Could you check a few things on this model? Use its own coordinates, in mm. Round coordinates to 2 decimals unless told otherwise and drop trailing zeros. Write each loop counter-clockwise with the first axis right and the second up, starting at its lowest first coordinate (ties: lowest second). Pieces come first, ordered by that corner, then holes. Notation, with made-up numbers: (75.5, 14) -> (110.5, 14) arc R13 cw to (110.5, 34) -> close; hole circle Ø1 at (5.25, -19.75). An arc over 180 degrees is marked (long way). One line per question, with ' | ' between items. Start each with the question number.
1. Thinking about a two-plate mould opening in Y: for faces 1 (the flat face through (-1, -1, 6)), 2 (the cylindrical face through (24.5, 7.1, 3)), 3 (the flat face through (-1, 35, 3)), which applies, released by +Y, released by -Y, zero draft, split by the parting line, or undercut?
2. If I drill on line 1 along Y through (x, z) = (-27, 2.35); line 2 along Y through (x, z) = (21.5, 2.3); line 3 along Y through (x, z) = (-26.5, 3.8), over which ranges is the centre line in solid material (lowest first)? Write a range as [from, to].
3. Imagine slicing it at D-D, the plane y = 7. List the corners of the cut face in (x, z) for me, and give its area (3 significant figures).
4. Imagine slicing it at A-A, the plane z = 3. List the corners of the cut face in (x, y) for me.
5. Imagine slicing it at C-C, the plane x = 0. List the corners of the cut face in (y, z) for me, and give its area (3 significant figures).
6. Imagine slicing it at B-B, the plane y = 30. List the corners of the cut face in (x, z) for me.
from build123d import *

# Parameters (mm, degrees)
SKETCH_1_W          = 80
SKETCH_1_H          = 60
SKETCH_1_R          = 7
EXTRUDE_1_DEPTH     = 6
SKETCH_2_R          = 3
SKETCH_2_R_2        = 2.555087711
CUT_EXTRUDE_1_DEPTH = 10


with BuildPart() as part:
    # 草图1 → 凸台-拉伸1 (new body)
    with BuildSketch(Plane.XY):
        with Locations((0, 5)):
            Rectangle(SKETCH_1_W, SKETCH_1_H)
        with Locations((0, 7)):
            Circle(SKETCH_1_R, mode=Mode.SUBTRACT)
    extrude(amount=EXTRUDE_1_DEPTH)

    # 草图2 → 切除-拉伸1 (cut)
    with BuildSketch(Plane(origin=(0, 0, 0), x_dir=(-1, 0, 0), z_dir=(0, 0, -1))):
        with Locations((-21.5, 7)):
            Circle(SKETCH_2_R)
        with Locations((26.5, 7)):
            Circle(SKETCH_2_R)
        with Locations((27, 30)):
            Circle(SKETCH_2_R_2)
        with Locations((27, -16)):
            Circle(SKETCH_2_R_2)
        with Locations((-25.052626778, -16)):
            Circle(SKETCH_2_R_2)
        with Locations((-25.052626778, 30)):
            Circle(SKETCH_2_R_2)
    extrude(amount=-CUT_EXTRUDE_1_DEPTH, mode=Mode.SUBTRACT)


solid = part.part
Geometry results:
1) face 1: zero draft | face 2: undercut | face 3: released by +Y
2) line 1: y = [-25, -18.56], [-13.44, 4.04], [9.96, 27.44], [32.56, 35] | line 2: y = [-25, 4], [10, 35] | line 3: y = [-25, -18.51], [-13.49, 4], [10, 27.49], [32.51, 35]
3) outline: (-40, 0) -> (-29.5, 0) -> (-29.5, 6) -> (-40, 6) -> close; (-23.5, 0) -> (-7, 0) -> (-7, 6) -> (-23.5, 6) -> close; (7, 0) -> (18.5, 0) -> (18.5, 6) -> (7, 6) -> close; (24.5, 0) -> (40, 0) -> (40, 6) -> (24.5, 6) -> close | area: 324 mm2
4) outline: (-40, -25) -> (40, -25) -> (40, 35) -> (-40, 35) -> close; hole circle Ø5.11 at (-27, -16); hole circle Ø5.11 at (-27, 30); hole circle Ø6 at (-26.5, 7); hole circle Ø14 at (0, 7); hole circle Ø6 at (21.5, 7); hole circle Ø5.11 at (25.05, -16); hole circle Ø5.11 at (25.05, 30)
5) outline: (-25, 0) -> (0, 0) -> (0, 6) -> (-25, 6) -> close; (14, 0) -> (35, 0) -> (35, 6) -> (14, 6) -> close | area: 276 mm2
6) outline: (-40, 0) -> (-29.56, 0) -> (-29.56, 6) -> (-40, 6) -> close; (-24.44, 0) -> (22.5, 0) -> (22.5, 6) -> (-24.44, 6) -> close; (27.61, 0) -> (40, 0) -> (40, 6) -> (27.61, 6) -> close
